Autodesk Inventor part; units mm, degrees
ref_plane "YZ Plane" through (0, 0, 0) normal (1, 0, 0) x (0, 1, 0)
ref_plane "XZ Plane" through (0, 0, 0) normal (0, 1, 0) x (-1, 0, 0)
ref_plane "XY Plane" through (0, 0, 0) normal (0, 0, 1) x (1, 0, 0)
sketch "Sketch1" plane through (0, 0, 0) normal (0, 0, 1) x (1, 0, 0)
  line L0 (0, 0) -> (-75, 0)
  line L1 (-75, 0) -> (-75, 75)
  line L2 (-75, 75) -> (0, 75)
  line L3 (0, 75) -> (0, 0)
  circle A0 centre (-5, 70) radius 2.65
  circle A1 centre (-70, 70) radius 2.65
  circle A2 centre (-5, 5) radius 2.65
  circle A3 centre (-70, 5) radius 2.65
  circle A4 centre (-37.5, 37.5) radius 25
  line L4 (-63, 61.5202) -> (-68, 61.5202)
  line L5 (-68, 61.5202) -> (-68, 11.5202)
  line L6 (-68, 11.5202) -> (-63, 11.5202)
  line L7 (-63, 11.5202) -> (-63, 61.5202)
  dimension "d0" = 75
  dimension "d1" = 75
  dimension "d2" = 5.3
  dimension "d3" = 5
  dimension "d4" = 5
  dimension "d7" = 65
  dimension "d10" = 65
  dimension "d26" = 50
  dimension "d29" = 50
  dimension "d30" = 5
  dimension "d31" = 25.5
  dimension "d32" = 37.5
extrude "Extrusion1" add sketch "Sketch1" along normal blind 2 contours L0 L1 L2 L3 | L7 L6 L5 L4
extrude "Extrusion2" add sketch "Sketch1" against normal blind 5 contours L7 L6 L5 L4
ref_plane "Work Plane1" through (-37.5, 37.5, 0) normal (1, 0, 0) x (0, 1, 0)
mirror "Mirror1" about plane through (-37.5, 37.5, 0) normal (1, 0, 0) of "Extrusion2"
fillet "Fillet2" radius 4 2 edges at (-68, 36.5202, 0) (-7, 36.5202, 0)
fillet "Fillet3" radius 4 4 edges at (0, 0, 1) (-75, 0, 1) (-75, 75, 1) (0, 75, 1)
equation "\"d1\" = d0"
equation "\"d4\" = d3"
equation "\"d7\" = d0 - 2 * d4"
equation "\"d10\" = d1 - 2 * d3"
equation "\"d32\" = 0.5 * d0"
properties part number "50x5 interface"
Source: CAD feature listing. Evaluate the final solid. Frame: model axes, mm. A direction names the side the tool comes from. Give positions to 0.01 mm unless a question says otherwise; leave off trailing zeros. Loops run counter-clockwise (first coordinate to the right, second up) from the corner with the lowest first, then second, coordinate; pieces in that order, holes last. Notation, with made-up numbers: (15, 41) - (37, 41) arc R16 ccw to (37, 51) - close; hole circle Ø11 at (21.25, -40). An arc over 180 degrees is marked (long way). Use CSV: the item, a comma, the result in double quotes.
1) Cut plane A-A (y = 37.5). Output: boundary loops of the cut face in (x, z), and give its area (3 significant figures).
Worked out:
outline,"(-75, 0) - (-72, 0) arc R4 cw to (-68, -4) - (-68, -5) - (-63, -5) - (-63, 0) - (-62.5, 0) - (-62.5, 2) - (-75, 2) - close; (-12.5, 0) - (-12, 0) - (-12, -5) - (-7, -5) - (-7, -4) arc R4 cw to (-3, 0) - (0, 0) - (0, 2) - (-12.5, 2) - close"
area,"107 mm^2"
2) Line query: line 1 (Y direction, x = -5, z = 0.6); line 2 (X direction, y = 38, z = -4); line 3 (Z direction, x = -44, y = 11). Output: solid intervals per line, ascending.
Worked out:
line 1,"y = 0 to 2.35, 7.65 to 67.35, 72.65 to 75"
line 2,"x = -68 to -63, -12 to -7"
line 3,"z = 0 to 2"
3) Cut plane C-C (y = 70). Output: boundary loops of the cut face in (x, z).
Worked out:
outline,"(-75, 0) - (-72.65, 0) - (-72.65, 2) - (-75, 2) - close; (-67.35, 0) - (-7.65, 0) - (-7.65, 2) - (-67.35, 2) - close; (-2.35, 0) - (0, 0) - (0, 2) - (-2.35, 2) - close"
4) Set-up query: faces 1 (the flat face through (0, 38, 1)), 2 (the flat face through (-12, 37, -2)), 3 (the flat face through (-9, 61.52, -2)). Return all of +Z, -Z, +X, -X, +Y, -Y with unobstructed straight access to the full face (end or side cutting, diameter ignored); none if empty.
Worked out:
face 1,"+Z, -Z, +X, +Y, -Y"
face 2,"-Z, +Y, -Y"
face 3,"-Z, +X, -X, +Y"
5) Cut plane B-B (x = -37.5). Output: boundary loops of the cut face in (y, z).
Worked out:
outline,"(0, 0) - (12.5, 0) - (12.5, 2) - (0, 2) - close; (62.5, 0) - (75, 0) - (75, 2) - (62.5, 2) - close"
6) Pin query (flat end, axial travel): P1, Ø4, axis at x = -6.5, z = -3.5, coming from the +Y side; P2, Ø1.5, axis at y = 37.5, z = -3, coming from the +X side; P3, Ø22.5, axis at x = -32.5, y = 49, coming from the -Z side; P4, Ø8.5, axis at x = -5, y = 70, coming from the -Z side. Return the tip coordinate at first contact, or that it passes through.
Worked out:
P1,"stops at y = 61.52"
P2,"stops at x = -6.6"
P3,"passes through"
P4,"stops at z = 0"
7) Mould query, pull axis Y, two halves, no side actions, for faces 4 (the flat face through (-66, 11.52, -2)), 5 (the flat face through (-63, 36, -2)), 6 (the cylindrical face through (-57.34, 52.71, 0.99)). Classes: +Y half, -Y half, draft (parallel to the pull), parting line (faces both ways), or undercut.
Worked out:
face 4,"-Y half"
face 5,"draft"
face 6,"undercut"
8) Cut plane D-D (x = -6). Output: boundary loops of the cut face in (y, z).
Worked out:
outline,"(0, 0) - (2.55, 0) - (2.55, 2) - (0, 2) - close; (7.45, 0) - (11.52, 0) - (11.52, -1.35) - (61.52, -1.35) - (61.52, 0) - (67.55, 0) - (67.55, 2) - (7.45, 2) - close; (72.45, 0) - (75, 0) - (75, 2) - (72.45, 2) - close"
